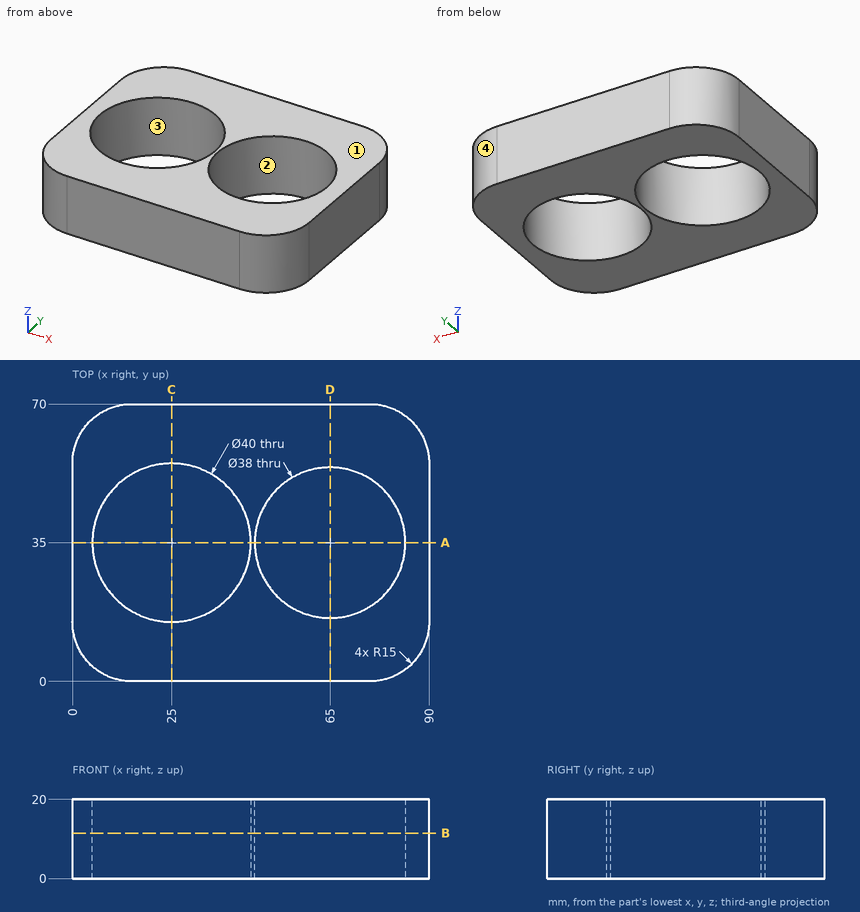
Verification items for this drawing (mm, ordinates from the low corner). Coordinates: 2 decimals unless noted, no trailing zeros. Write each loop counter-clockwise with the first axis right and the second up, starting at its lowest first coordinate (ties: lowest second). Pieces come first, ordered by that corner, then holes. Notation, with made-up numbers: M -6,61 L 13,61 A20 cw 13,70 Z; hole C 61.25,42.25 d11. An arc over 180 degrees is marked long. Use one line per item in the form item = value. Start each with the question number.
1) Section check A-A on y = 35. Enter the section's corners in (x, z), and give its area (3 significant figures).
2) Section check B-B on z = 11.5. Enter the section's corners in (x, y).
3) Release check for a two-part mould opening along Y. For the marked faces 1, 2, 3 and 4 record: pulls with the +Y half, pulls with the -Y half, needs draft (parallel to the pull), parting line crosses it, or undercut.
4) Section check C-C on x = 25. Enter the section's corners in (y, z).
5) Section check D-D on x = 65. Enter the section's corners in (y, z).
6) Thickness scan on probe 1 along X at (y, z) = (20.5, 15.5); probe 2 along X at (y, z) = (40, 5.5); probe 3 along Y at (x, z) = (65, 8). Record the ranges inside material, lowest first. Write a range as from..to.
Responses:
q1.outline = M 0,0 L 5,0 L 5,20 L 0,20 Z; M 45,0 L 46,0 L 46,20 L 45,20 Z; M 84,0 L 90,0 L 90,20 L 84,20 Z
q1.area = 240 mm2
q2.outline = M 0,15 A15 ccw 15,0 L 75,0 A15 ccw 90,15 L 90,55 A15 ccw 75,70 L 15,70 A15 ccw 0,55 Z; hole C 25,35 d40; hole C 65,35 d38
q3.face_1 = needs draft
q3.face_2 = undercut
q3.face_3 = undercut
q3.face_4 = pulls with the +Y half
q4.outline = M 0,0 L 15,0 L 15,20 L 0,20 Z; M 55,0 L 70,0 L 70,20 L 55,20 Z
q5.outline = M 0,0 L 16,0 L 16,20 L 0,20 Z; M 54,0 L 70,0 L 70,20 L 54,20 Z
q6.probe_1 = 0..11.23, 38.77..52.72, 77.28..90
q6.probe_2 = 0..5.64, 44.36..46.67, 83.33..90
q6.probe_3 = 0..16, 54..70
